Verification items for the finished model (mm, model axes). Round coordinates to 2 decimals unless told otherwise and drop trailing zeros. Loops run counter-clockwise (first coordinate to the right, second up) from the corner with the lowest first, then second, coordinate; pieces in that order, holes last. Notation, with made-up numbers: (72, 47.25) -> (129, 47.25) arc R30 ccw to (129, 84.25) -> close; hole circle Ø10 at (-18, 81.25). An arc over 180 degrees is marked (long way). Write item = value, one per line.
```python
from build123d import *

# Parameters (mm, degrees)
F0_R     = 200
F1_DEPTH = 225
F2_W     = 460
F2_H     = 450
F3_DEPTH = 230


with BuildPart() as f1:
    # F0 (on Top) → F1 (new body, symmetric)
    with BuildSketch(Plane.XY):
        Circle(F0_R)
    extrude(amount=F1_DEPTH, both=True)


with BuildPart() as f3:
    # F2 (on Front) → F3 (new body)
    with BuildSketch(Plane.XZ):
        Rectangle(F2_W, F2_H)
    extrude(amount=F3_DEPTH)

    # F4: cut F1
    add(f1.part, mode=Mode.SUBTRACT)


solid = f3.part
```
(1) Material ranges on probe 1 along X at (y, z) = (-133, -50.5); probe 2 along X at (y, z) = (-147, 43); probe 3 along Y at (x, z) = (17, -120), recorded low to high. Write a range as from..to.
Filled sheet:
probe_1 = -230..-149.37, 149.37..230
probe_2 = -230..-135.61, 135.61..230
probe_3 = -230..-199.28
(2) Sectioned sample at C-C, the plane y = -172. Record the cut outline in (x, z), and give its area (3 significant figures).
Filled sheet:
outline = (-230, -225) -> (-102.06, -225) -> (-102.06, 225) -> (-230, 225) -> close; (102.06, -225) -> (230, -225) -> (230, 225) -> (102.06, 225) -> close
area = 115,000 mm2
(3) Go/stop test with a flat-tipped pin: pin 1 Ø2 at (x, z) = (-116, -141.5) entering from +Y. Record where the tip stops, or that it passes through.
Filled sheet:
pin_1 = -162.21
(4) Draft check along X on faces 1 (the face through (215, 0, 3)), 2 (the face through (-4.4, -199.95, 3.15)), 3 (the face through (-230, -113, -3)), 4 (the face through (230, -113, -3)). Enter one of: released by +X, released by -X, zero draft, split by the parting line, or undercut.
Filled sheet:
face_1 = zero draft
face_2 = undercut
face_3 = released by -X
face_4 = released by +X
(5) Sectioned sample at A-A, the plane y = -92. Record the cut outline in (x, z), and give its area (3 significant figures).
Filled sheet:
outline = (-230, -225) -> (-177.58, -225) -> (-177.58, 225) -> (-230, 225) -> close; (177.58, -225) -> (230, -225) -> (230, 225) -> (177.58, 225) -> close
area = 47,200 mm2
(6) Sectioned sample at B-B, the plane z = -140. Record the cut outline in (x, y).
Filled sheet:
outline = (-230, -230) -> (230, -230) -> (230, 0) -> (200, 0) arc R200 cw to (-200, 0) -> (-230, 0) -> close
(7) Sectioned sample at D-D, the plane x = 0. Record the cut outline in (y, z).
Filled sheet:
outline = (-230, -225) -> (-200, -225) -> (-200, 225) -> (-230, 225) -> close
